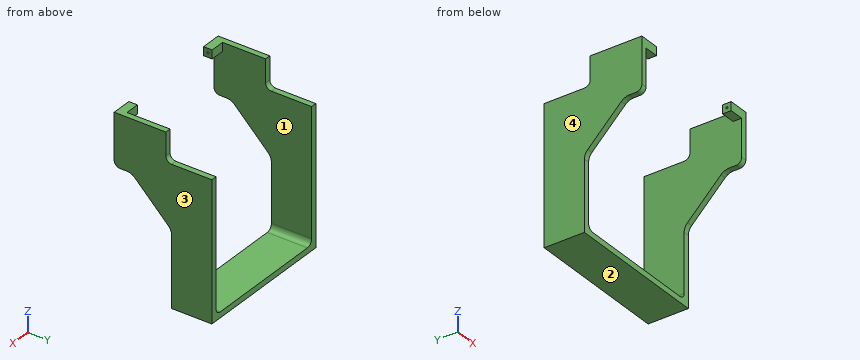
```python
from build123d import *

# Parameters (mm, degrees)
SKETCH_1_W          = 250
SKETCH_1_H          = 170
EXTRUDE_1_DEPTH     = 10
SKETCH_2_W          = 10
SKETCH_2_H          = 170
EXTRUDE_2_DEPTH     = 280
SKETCH_3_W          = 15
SKETCH_3_H          = 15
EXTRUDE_3_DEPTH     = 25
SKETCH_4_W          = 15
SKETCH_4_H          = 15
EXTRUDE_4_DEPTH     = 25
SKETCH_5_R          = 1.7
CUT_EXTRUDE_1_DEPTH = 5
CUT_EXTRUDE_START   = -5
SKETCH_6_R          = 1.7
CUT_EXTRUDE_2_DEPTH = 5
SKETCH_7_W          = 250
SKETCH_7_H          = 100
CUT_EXTRUDE_3_DEPTH = 200
SKETCH_8_W          = 250
SKETCH_8_H          = 80
CUT_EXTRUDE_4_DEPTH = 50
FILLET_1_R          = 10
CHAMFER_2_SIZE      = 70
FILLET_3_R          = 20


with BuildPart() as part:
    # 草图1 → 凸台-拉伸1 (new body)
    with BuildSketch(Plane.XY):
        Rectangle(SKETCH_1_W, SKETCH_1_H)
    extrude(amount=EXTRUDE_1_DEPTH)

    # 草图2 → 凸台-拉伸2 (add)
    with BuildSketch(Plane.XY.offset(10)):
        with Locations((-120, 0)):
            Rectangle(SKETCH_2_W, SKETCH_2_H)
        with Locations((120, 0)):
            Rectangle(SKETCH_2_W, SKETCH_2_H)
    extrude(amount=EXTRUDE_2_DEPTH)

    # 草图3 → 凸台-拉伸3 (add)
    with BuildSketch(Plane(origin=(-115, 0, 0), x_dir=(0, 0, -1), z_dir=(1, 0, 0))):
        with Locations((-282.5, -77.5)):
            Rectangle(SKETCH_3_W, SKETCH_3_H)
    extrude(amount=EXTRUDE_3_DEPTH)

    # 草图4 → 凸台-拉伸4 (add)
    with BuildSketch(Plane.ZY.offset(-115)):
        with Locations((282.5, -77.5)):
            Rectangle(SKETCH_4_W, SKETCH_4_H)
    extrude(amount=EXTRUDE_4_DEPTH)

    # 草图5 → 切除-拉伸1 (cut)
    with BuildSketch(Plane.ZY.offset(-90)):
        with Locations(Location((282.5, -77.5, 0), (0, 0, 270))):
            Circle(SKETCH_5_R)
    extrude(amount=-CUT_EXTRUDE_1_DEPTH, mode=Mode.SUBTRACT)

    # 草图6 → 切除-拉伸2 (cut)
    with BuildSketch(Plane(origin=(-90, 0, 0), x_dir=(0, 0, -1), z_dir=(1, 0, 0)).offset(CUT_EXTRUDE_START)):
        with Locations(Location((-282.5, -77.5, 0), (0, 0, 270))):
            Circle(SKETCH_6_R)
    extrude(amount=CUT_EXTRUDE_2_DEPTH, mode=Mode.SUBTRACT)

    # 草图7 → 切除-拉伸3 (cut)
    with BuildSketch(Plane(origin=(0, 0, 0), x_dir=(-1, 0, 0), z_dir=(0, 0, -1))):
        with Locations((0, -35)):
            Rectangle(SKETCH_7_W, SKETCH_7_H)
    extrude(amount=-CUT_EXTRUDE_3_DEPTH, mode=Mode.SUBTRACT)

    # 草图8 → 切除-拉伸4 (cut)
    with BuildSketch(Plane.XY.offset(290)):
        with Locations((0, 45)):
            Rectangle(SKETCH_8_W, SKETCH_8_H)
    extrude(amount=-CUT_EXTRUDE_4_DEPTH, mode=Mode.SUBTRACT)

    # 圆角1
    fillet_1_edges = [part.edges().sort_by_distance(p)[0] for p in [
        (120, 5, 240),
        (-120, 5, 240),
        (115, 50, 10),
        (-115, 50, 10),
        (120, -85, 200),
        (-120, -85, 200),
    ]]
    fillet(fillet_1_edges, radius=FILLET_1_R)

    # 倒角2
    chamfer_2_edges = [part.edges().sort_by_distance(p)[0] for p in [
        (120, 15, 200),
        (-120, 15, 200),
    ]]
    chamfer(chamfer_2_edges, length=CHAMFER_2_SIZE)

    # 圆角3
    fillet_3_edges = [part.edges().sort_by_distance(p)[0] for p in [
        (120, -55, 200),
        (-120, 15, 130),
        (120, 15, 130),
        (-120, -55, 200),
    ]]
    fillet(fillet_3_edges, radius=FILLET_3_R)


solid = part.part
```
CAD build for the part. Positions are in the model's coordinates, mm. Face numbers are marked on the shaded views. Coordinates: 2 decimals unless noted, no trailing zeros. Order: outer loops, then holes, each group sorted by start corner. A loop starts at its lowest first (then second) coordinate and runs counter-clockwise, first axis right, second up.
(1) Saw through at B-B, the plane y = -22. Write the cut outline in (x, z), and give its area (3 significant figures).
Solution:
outline: (-125, 167) - (-115, 167) - (-115, 290) - (-125, 290) - close; (115, 167) - (125, 167) - (125, 290) - (115, 290) - close
area: 2,460 mm2
(2) Saw through at A-A, the plane z = 53.5. Write the cut outline in (x, y), and give its area (3 significant figures).
Solution:
outline: (-125, 15) - (-115, 15) - (-115, 85) - (-125, 85) - close; (115, 15) - (125, 15) - (125, 85) - (115, 85) - close
area: 1,400 mm2
(3) Saw through at D-D, the plane x = 15. Write the cut outline in (y, z).
Solution:
outline: (15, 0) - (85, 0) - (85, 10) - (15, 10) - close
(4) Drill centre lines: L1, parallel to Z at x = 91.1, y = -77.5; L2, parallel to Z at x = 93, y = -77; L3, parallel to Y at x = -91.55, z = 282.5. Where is each one in solid material? Low to high.
Solution:
L1: z = 275 to 280.8, 284.2 to 290
L2: z = 275 to 280.88, 284.12 to 290
L3: y = -85 to -79.2, -75.8 to -70
(5) Pin check, flat tips, straight feed: pin 1 Ø11 at (x, z) = (-118, 269) entering from +Y; pin 2 Ø4.5 at (x, y) = (106.5, -78.5) entering from -Z; pin 3 Ø3 at (x, y) = (-120.5, -66.5) entering from -Z. Stop position of each tip, or through.
Solution:
pin 1: stops at y = 5
pin 2: stops at z = 275
pin 3: stops at z = 200
(6) Saw through at C-C, the plane y = 49. Write the cut outline in (x, z).
Solution:
outline: (-125, 0) - (125, 0) - (125, 240) - (115, 240) - (115, 20) arc R10 cw to (105, 10) - (-105, 10) arc R10 cw to (-115, 20) - (-115, 240) - (-125, 240) - close
(7) Mould opens along X. For the marked faces 1, 2, 3 and 4 say: released by +X, released by -X, zero draft, split by the parting line, or undercut.
Solution:
face 1: undercut
face 2: zero draft
face 3: released by +X
face 4: released by -X
